Geometry: final body of the model. Coordinates: model frame, mm. A direction names the side the tool comes from. Give positions to 0.01 mm unless a question says otherwise; leave off trailing zeros. Loops run counter-clockwise (first coordinate to the right, second up) from the corner with the lowest first, then second, coordinate; pieces in that order, holes last. Notation, with made-up numbers: (41.5, 89.25) - (88.5, 89.25) arc R18 ccw to (88.5, 107.25) - close; hole circle Ø4 at (46, -39.5). An arc over 180 degrees is marked (long way). Answer in a Markdown table with one row per item.
from build123d import *

# Parameters (mm, degrees)
EXTRUDE_1_DEPTH     = 37
CUT_EXTRUDE_1_DEPTH = 33
SKETCH_3_W          = 15
SKETCH_3_H          = 1.9
EXTRUDE_2_DEPTH     = 5
SKETCH_4_R          = 2
CUT_EXTRUDE_2_DEPTH = 10
SKETCH_5_R          = 1.5
CUT_EXTRUDE_3_DEPTH = 47.596673701


with BuildPart() as part:
    # 草图1 → 凸台-拉伸1 (new body)
    with BuildSketch(Plane(origin=(0, 0, 0), x_dir=(1, 0, 0), z_dir=(0, 1, 0))):
        with BuildLine():
            Line((-3.5, 15), (13.5, 15))
            Line((13.5, 15), (13.5, -15))
            Line((13.5, -15), (-13.5, -15))
            Line((-13.5, -15), (-13.5, 5))
            ThreePointArc((-13.5, 5), (-10.571067812, 12.071067812), (-3.5, 15))
        make_face()
    extrude(amount=EXTRUDE_1_DEPTH)

    # 草图2 → 切除-拉伸1 (cut)
    with BuildSketch(Plane(origin=(0, 0, 0), x_dir=(1, 0, 0), z_dir=(0, 1, 0))):
        with BuildLine():
            Line((-11.499999995, -15), (13.5, -15))
            Line((13.5, -15), (13.5, 10))
            Line((13.5, 10), (-1.5, 10))
            Line((-1.5, 10), (-1.5, 15))
            Line((-1.5, 15), (-13.5, 15))
            Line((-13.5, 15), (-13.5, -13))
            ThreePointArc((-13.5, -13), (-11.5, -11), (-9.5, -13))
            ThreePointArc((-9.5, -13), (-10.085786436, -14.414213561), (-11.499999995, -15))
        make_face()
        with BuildLine():
            Line((-13.5, -15), (-11.499999995, -15))
            ThreePointArc((-11.499999995, -15), (-12.914213561, -14.414213564), (-13.5, -13))
            Line((-13.5, -13), (-13.5, -15))
        make_face()
    extrude(amount=CUT_EXTRUDE_1_DEPTH, mode=Mode.SUBTRACT)

    # 草图3 → 凸台-拉伸2 (add)
    with BuildSketch(Plane.XZ):
        with Locations((6, -12.15)):
            Rectangle(SKETCH_3_W, SKETCH_3_H)
    extrude(amount=EXTRUDE_2_DEPTH)

    # 草图4 → 切除-拉伸2 (cut)
    with BuildSketch(Plane.XZ.offset(-33)):
        with Locations(Location((1.4, 1.9, 0), (0, 0, 270))):
            Circle(SKETCH_4_R)
    extrude(amount=-CUT_EXTRUDE_2_DEPTH, mode=Mode.SUBTRACT)

    # 草图5 → 切除-拉伸3 (cut, through all)
    with BuildSketch(Plane(origin=(0, 37, 0), x_dir=(1, 0, 0), z_dir=(0, 1, 0))):
        with Locations(Location((-7.1, 6.6, 0), (0, 0, 270))):
            Circle(SKETCH_5_R)
        with Locations(Location((9.9, -10.4, 0), (0, 0, 270))):
            Circle(SKETCH_5_R)
    extrude(amount=-CUT_EXTRUDE_3_DEPTH, mode=Mode.SUBTRACT)


solid = part.part
Q1. Draft query along X for faces 4 (the cylindrical face through (-10.65, 34.97, -11.99)), 5 (the flat face through (6, -2, -13.1)), 6 (the cylindrical face through (-5.835, 35.028, -5.794)). Return one class per face: pulls with the +X half, pulls with the -X half, needs draft (parallel to the pull), parting line crosses it, or undercut.
Check values:
| item | result |
|---|---|
| face 4 | pulls with the -X half |
| face 5 | needs draft |
| face 6 | undercut |
Q2. Cut plane C-C (z = 1.9). Output: boundary loops of the cut face in (x, y), and give its area (3 significant figures).
Check values:
| item | result |
|---|---|
| outline | (-13.5, 33) - (-0.6, 33) - (-0.6, 37) - (-13.5, 37) - close; (3.4, 33) - (13.5, 33) - (13.5, 37) - (3.4, 37) - close |
| area | 92.0 mm² |
Q3. Reachability of faces 1 (the flat face through (6, 0, -14)), 2 (the flat face through (-13.1, 33, 14.5)), 3 (the flat face through (-1.5, 14, -12)) from +Z, -Z, +X, -X, +Y, -Y: full face, straight path, thin tool, end or side. Return the list, or none.
Check values:
| item | result |
|---|---|
| face 1 | -Z, +X, -X, -Y |
| face 2 | +Z, -X, -Y |
| face 3 | +Z, -Z, -X, -Y |
Q4. Cut plane B-B (x = 1.4). Output: boundary loops of the cut face in (y, z), and give its area (4 significant figures).
Check values:
| item | result |
|---|---|
| outline | (-5, -13.1) - (0, -13.1) - (0, -15) - (37, -15) - (37, -0.1) - (33, -0.1) - (33, -10) - (0, -10) - (0, -11.2) - (-5, -11.2) - close; (33, 3.9) - (37, 3.9) - (37, 15) - (33, 15) - close |
| area | 278.5 mm² |
Q5. Cut plane A-A (y = 10.5). Output: boundary loops of the cut face in (x, z), and give its area (3 significant figures).
Check values:
| item | result |
|---|---|
| outline | circle Ø4 at (-11.5, 13); (-1.5, -15) - (13.5, -15) - (13.5, -10) - (-1.5, -10) - close |
| area | 87.6 mm² |
Q6. Cut plane D-D (x = 9.9). Output: boundary loops of the cut face in (y, z), and give its area (4 significant figures).
Check values:
| item | result |
|---|---|
| outline | (-5, -13.1) - (0, -13.1) - (0, -15) - (37, -15) - (37, 8.9) - (33, 8.9) - (33, -10) - (0, -10) - (0, -11.2) - (-5, -11.2) - close; (33, 11.9) - (37, 11.9) - (37, 15) - (33, 15) - close |
| area | 282.5 mm² |
Q7. First-contact query: pin 1 (2 mm diameter, centred on x = 8.5, y = 14, fed in from +Z); pin 2 (2 mm diameter, centred on x = 9, z = -14.5, fed in from -Y); pin 3 (4 mm diameter, centred on x = 3.5, y = -2.5, fed in from -Z). Flat tips, straight axial feed; report the tip coordinate or a pass-through.
Check values:
| item | result |
|---|---|
| pin 1 | z = -10 |
| pin 2 | y = 0 |
| pin 3 | z = -13.1 |
Q8. Material intervals for line 1 along X through (y, z) = (33.9, 10.4); line 2 along X through (y, z) = (34.45, 1.9); line 3 along Y through (x, z) = (8.75, -7), sorted ascending.
Check values:
| item | result |
|---|---|
| line 1 | -13.5 to 8.4, 11.4 to 13.5 |
| line 2 | -13.5 to -0.6, 3.4 to 13.5 |
| line 3 | 33 to 37 |
